Check sheet for the modelled part. Datum: model origin and axes. Units: mm. Face numbers are marked on the shaded views. A direction names the side the tool comes from. Coordinates: 2 decimals unless noted, no trailing zeros. Loops run counter-clockwise (first coordinate to the right, second up) from the corner with the lowest first, then second, coordinate; pieces in that order, holes last. Notation, with made-up numbers: M -8.5,-9 L 39.5,-9 A4 ccw 39.5,-3 Z; hole C -6,42.25 d7. An arc over 180 degrees is marked long. Write each question's results on one line, items separated by ' | '. Start each with the question number.
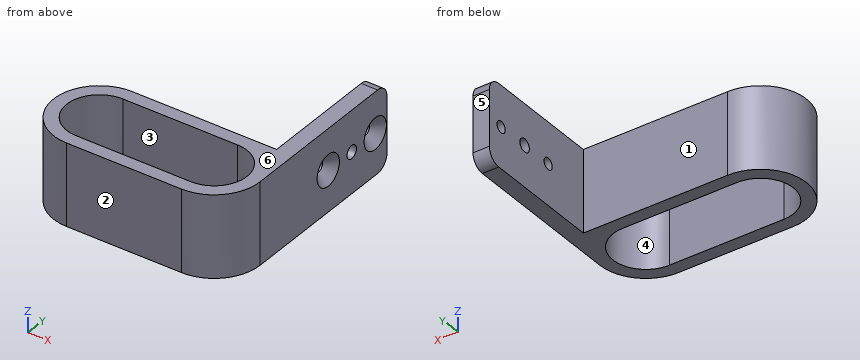
from build123d import *

# Parameters (mm, degrees)
PAD_DEPTH       = 25
FILLET_R        = 4
SKETCH001_R     = 2
SKETCH001_R_2   = 1.75
POCKET_DEPTH    = 63.001
CHAMFER_SIZE    = 3
CHAMFER001_SIZE = 3


with BuildPart() as part:
    # Sketch → Pad (new body)
    with BuildSketch(Plane.XY):
        with BuildLine():
            ThreePointArc((-17.5, 14), (-31.5, 0), (-17.5, -14))
            Line((-17.5, -14), (17.5, -14))
            ThreePointArc((17.5, -14), (27.399495, -9.899495), (31.5, 0))
            Line((31.5, 0), (31.5, 54))
            Line((26.5, 54), (31.5, 54))
            Line((26.5, 14), (26.5, 54))
            Line((-17.5, 14), (26.5, 14))
        make_face()
        with BuildLine():
            ThreePointArc((-17.5, 10), (-27.5, 0), (-17.5, -10))
            Line((-17.5, -10), (17.5, -10))
            ThreePointArc((17.5, -10), (27.5, 0), (17.5, 10))
            Line((-17.5, 10), (17.5, 10))
        make_face(mode=Mode.SUBTRACT)
    extrude(amount=PAD_DEPTH)

    # Fillet
    fillet_edges = [part.edges().sort_by_distance(p)[0] for p in [
        (29, 54, 0),
        (29, 54, 25),
    ]]
    fillet(fillet_edges, radius=FILLET_R)

    # Sketch001 (on Face8 of Fillet) → Pocket (cut, through all)
    with BuildSketch(Plane.YZ.offset(31.5)):
        with Locations((39, 12.5)):
            Circle(SKETCH001_R)
        with Locations((49, 12.5)):
            Circle(SKETCH001_R_2)
        with Locations((29, 12.5)):
            Circle(SKETCH001_R_2)
    extrude(amount=-POCKET_DEPTH, mode=Mode.SUBTRACT)

    # Chamfer
    chamfer_edges = [part.edges().sort_by_distance(p)[0] for p in [
        (31.5, 27.25, 12.5),
    ]]
    chamfer(chamfer_edges, length=CHAMFER_SIZE)

    # Chamfer001
    chamfer001_edges = [part.edges().sort_by_distance(p)[0] for p in [
        (31.5, 47.25, 12.5),
    ]]
    chamfer(chamfer001_edges, length=CHAMFER001_SIZE)


solid = part.part
1) Section check A-A (z = 12.5). Enter the section's corners in (x, y).
2) Section check D-D (z = 22.75). Enter the section's corners in (x, y), then the cut area to 3 significant figures.
3) Release check for a two-part mould opening along Y. For the marked faces 4, 5 and 6 record: +Y half, -Y half, draft (parallel to the pull), parting line (faces both ways), or undercut.
4) Set-up check for the marked faces 1, 2 and 3: record each of +Z, -Z, +X, -X, +Y, -Y from which the full face is reachable in a straight line by a thin tool's end or side.
5) Section check C-C (x = -10). Enter the section's corners in (y, z), then the cut area to 3 significant figures.
6) Section check B-B (y = 39). Enter the section's corners in (x, z), then the cut area to 3 significant figures.
7) Gauge pin test, flat ends, axial feed: P1, Ø7.5, axis at x = -7, z = 10, coming from the +Y side; P2, Ø5.5, axis at y = 29, z = 12.5, coming from the +X side; P3, Ø1.5, axis at y = 18, z = 20.5, coming from the -X side; P4, Ø2.5, axis at y = 39, z = 12.5, coming from the -X side. Record the tip position at first contact, or that the pin passes through.
8) Thickness scan on probe 1 along Y at (x, z) = (-13, 10.25); probe 2 along Z at (x, y) = (27.05, 29); probe 3 along Z at (x, y) = (30, 39). Record the ranges inside material, lowest first.
Return value:
1) outline: M -17.5,-14 L 17.5,-14 A14 ccw 31.5,0 L 31.5,24.25 L 28.5,27.25 L 26.5,27.25 L 26.5,14 L -17.5,14 A14 ccw Z; M 26.5,30.75 L 28.5,30.75 L 31.5,33.75 L 31.5,37 L 26.5,37 Z; M 26.5,41 L 31.5,41 L 31.5,44.25 L 28.5,47.25 L 26.5,47.25 Z; M 26.5,50.75 L 28.5,50.75 L 31.5,53.75 L 31.5,54 L 26.5,54 Z; hole M -17.5,-10 L 17.5,-10 A10 ccw 17.5,10 L -17.5,10 A10 ccw Z
2) outline: M -17.5,-14 L 17.5,-14 A14 ccw 31.5,0 L 31.5,53.6 L 26.5,53.6 L 26.5,14 L -17.5,14 A14 ccw Z; hole M -17.5,-10 L 17.5,-10 A10 ccw 17.5,10 L -17.5,10 A10 ccw Z | area: 822 mm2
3) face 4: undercut | face 5: +Y half | face 6: draft
4) face 1: +Z, -Z, -X, +Y | face 2: +Z, -Z, +X, -X, -Y | face 3: +Z, -Z
5) outline: M -14,0 L -10,0 L -10,25 L -14,25 Z; M 10,0 L 14,0 L 14,25 L 10,25 Z | area: 200 mm2
6) outline: M 26.5,0 L 31.5,0 L 31.5,10.5 L 26.5,10.5 Z; M 26.5,14.5 L 31.5,14.5 L 31.5,25 L 26.5,25 Z | area: 105 mm2
7) P1: stops at y = 14 | P2: stops at x = 29.5 | P3: stops at x = 26.5 | P4: passes through
8) probe 1: y = -14 to -10, 10 to 14 | probe 2: z = 0 to 10.75, 14.25 to 25 | probe 3: z = 0 to 10.5, 14.5 to 25
